Check sheet for the modelled part. Datum: model origin and axes. Units: mm. Face numbers are marked on the shaded views. Coordinates: 2 decimals unless noted, no trailing zeros. Write each loop counter-clockwise with the first axis right and the second up, starting at its lowest first coordinate (ties: lowest second). Pieces come first, ordered by that corner, then holes. Notation, with made-up numbers: M 15,33 L 47,33 A21 cw 47,44 Z; hole C 26,82 d7. An arc over 180 degrees is marked long. Answer as CSV lines item,"result". Start each with the question number.
Q1. Sectioned sample at A-A, the plane y = 12. Record the cut outline in (x, z).
Q2. Mould release check, pull along X, two halves, no side actions. Record for the marked faces 1 and 2: pulls with the +X half, pulls with the -X half, needs draft (parallel to the pull), parting line crosses it, or undercut.
Q3. Sectioned sample at C-C, the plane y = 61. Record the cut outline in (x, z), then the cut area to 3 significant figures.
Q4. Sectioned sample at D-D, the plane z = 18. Record the cut outline in (x, y).
Q5. Depth check by flat-ended pin: pin 1 Ø4.5 at (y, z) = (80.98, 9.12) entering from -X; pin 2 Ø0.5 at (x, y) = (1, 47.5) entering from -Z; pin 3 Ø3 at (x, z) = (-2.5, 9.5) entering from -Y; pin 4 Ø0.8 at (x, z) = (1, 6) entering from -Y. Enter the tip coordinate at first touch or a pass-through.
Q6. Thickness scan on line 1 along Y through (x, z) = (0.55, 10.5); line 2 along X through (y, z) = (62, 13.25); line 3 along Y through (x, z) = (0.7, 3.25). Record the ranges inside material, lowest first. Write a range as from..to.
Q7. Sectioned sample at B-B, the plane z = 4.75. Record the cut outline in (x, y), then the cut area to 3 significant figures.
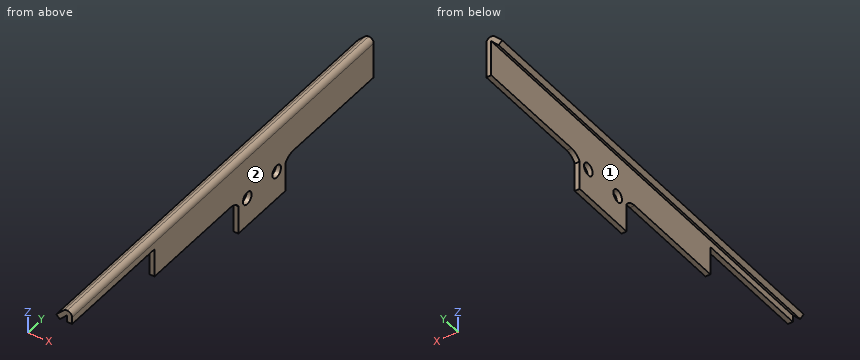
from build123d import *

# Parameters (mm, degrees)
F0_W      = 139.446
F0_H      = 24.0284
F1_DEPTH  = 1.5748
F2_R      = 2.5273
F2_R_2    = 1.9812
F3_DEPTH  = 25.4
F4_W      = 76.8604
F4_H      = 9.1186
F4_W_2    = 40.894
F5_DEPTH  = 25.4
F7_DEPTH  = 25.4
F9_DEPTH  = 139.447
F10_DEPTH = 139.446
F11_R     = 2.5273
F12_DEPTH = 25.4
F14_DEPTH = 1.5748
F15_DEPTH = 25.4


# Not quite as in the source:
# - ends of sketch curves that miss each other by under 0.0002 mm in the source are joined


with BuildPart() as f1:
    # F0 (on Right) → F1 (new body)
    with BuildSketch(Plane.YZ):
        with Locations((69.723, 12.0142)):
            Rectangle(F0_W, F0_H)
    extrude(amount=F1_DEPTH)

    # F2 (on face) → F3 (cut)
    with BuildSketch(Plane.YZ.offset(1.5748)):
        with Locations((7.9502, 14.6812)):
            Circle(F2_R)
        with Locations((80.9752, 9.1186)):
            Circle(F2_R_2)
        with Locations((94.5642, 9.1186)):
            Circle(F2_R_2)
    extrude(amount=-F3_DEPTH, mode=Mode.SUBTRACT)

    # F4 (on face) → F5 (cut)
    with BuildSketch(Plane.YZ.offset(1.5748)):
        with Locations((38.4302, 4.5593)):
            Rectangle(F4_W, F4_H)
        with Locations((118.999, 4.5593)):
            Rectangle(F4_W_2, F4_H)
    extrude(amount=-F5_DEPTH, mode=Mode.SUBTRACT)

    # F6 (on face) → F7 (cut)
    with BuildSketch(Plane.YZ.offset(1.5748)):
        with BuildLine():
            ThreePointArc((102.3057040906, 11.0998), (104.4279345117, 10.5741090514), (106.0594081813, 9.1186))
            Line((106.0594081813, 9.1186), (139.446, 9.1186))
            Line((139.446, 9.1186), (139.446, 11.0998))
            Line((139.446, 11.0998), (102.3057040906, 11.0998))
        make_face()
        with BuildLine():
            Line((98.552, 9.1186), (106.0594081813, 9.1186))
            ThreePointArc((106.0594081813, 9.1186), (104.4279345117, 10.5741090514), (102.3057040906, 11.0998))
            ThreePointArc((102.3057040906, 11.0998), (100.1834736696, 10.5741090514), (98.552, 9.1186))
        make_face()
        with BuildLine():
            ThreePointArc((25.0643040906, 9.1186), (23.4328304559, 10.574109033), (21.3106000788, 11.0998))
            ThreePointArc((21.3106000788, 11.0998), (19.1883696138, 10.5741090698), (17.5568959094, 9.1186))
            Line((17.5568959094, 9.1186), (25.0643040906, 9.1186))
        make_face()
        with BuildLine():
            ThreePointArc((69.3529918187, 9.1186), (70.9844654883, 10.5741090514), (73.1066959094, 11.0998))
            Line((73.1066959094, 11.0998), (21.3106000788, 11.0998))
            ThreePointArc((21.3106000788, 11.0998), (23.4328304559, 10.574109033), (25.0643040906, 9.1186))
            Line((25.0643040906, 9.1186), (69.3529918187, 9.1186))
        make_face()
        with BuildLine():
            ThreePointArc((76.8604, 9.1186), (75.2289263304, 10.5741090514), (73.1066959094, 11.0998))
            ThreePointArc((73.1066959094, 11.0998), (70.9844654883, 10.5741090514), (69.3529918187, 9.1186))
            Line((69.3529918187, 9.1186), (76.8604, 9.1186))
        make_face()
    extrude(amount=-F7_DEPTH, mode=Mode.SUBTRACT)

    # F8 (on face) → F9 (cut, through all)
    with BuildSketch(Plane.XZ):
        with BuildLine():
            Line((1.5748, 24.0284), (0, 24.0284))
            ThreePointArc((0, 24.0284), (1.1139794542, 23.562560882), (1.5748, 22.4465026135))
            Line((1.5748, 22.4465026135), (1.5748, 24.0284))
        make_face()
    extrude(amount=-F9_DEPTH, mode=Mode.SUBTRACT)

    # F8 (on face) → F10 (join)
    with BuildSketch(Plane.XZ):
        with BuildLine():
            Line((0, 24.0284), (0, 22.4536))
            Line((0, 22.4536), (0, 22.4465026135))
            Line((0, 22.4465026135), (1.5748, 22.4465026135))
            ThreePointArc((1.5748, 22.4465026135), (1.1139794542, 23.562560882), (0, 24.0284))
        make_face()
        with BuildLine():
            Line((-1.2264893587, 23.4542141594), (-0.0070973865, 22.4465026135))
            Line((-0.0070973865, 22.4465026135), (0, 22.4536))
            Line((0, 22.4536), (0, 24.0284))
            ThreePointArc((0, 24.0284), (-0.6777928151, 23.8791808689), (-1.2264893587, 23.4542141594))
        make_face()
        Polygon((-3.4544, 21.226303518), (-2.340848241, 20.112751759), (-0.0070973865, 22.4465026135), (-1.2264893587, 23.4542141594), align=None)
    extrude(amount=-F10_DEPTH)

    # F11 (on face) → F12 (cut)
    with BuildSketch(Plane(origin=(0, 0, 0), x_dir=(0, -1, 0), z_dir=(-1, 0, 0))):
        with BuildLine():
            Line((-17.5568959094, 9.1186), (0, 9.1186))
            Line((0, 9.1186), (0, 20.2311))
            Line((0, 20.2311), (-38.1, 20.2311))
            Line((-38.1, 20.2311), (-38.1, 11.0998))
            Line((-38.1, 11.0998), (-21.3106000788, 11.0998))
            ThreePointArc((-21.3106000788, 11.0998), (-19.1883696138, 10.5741090698), (-17.5568959094, 9.1186))
        make_face()
        with Locations((-7.9502, 14.6812)):
            Circle(F11_R, mode=Mode.SUBTRACT)
    extrude(amount=-F12_DEPTH, mode=Mode.SUBTRACT)


with BuildPart() as f14:
    # F13 (on Right) → F14 (new body, through all)
    with BuildSketch(Plane.YZ):
        with BuildLine():
            Line((38.1, 20.2311), (0, 20.2311))
            Line((0, 20.2311), (0, 0))
            Line((0, 0), (16.764, 0))
            Line((16.764, 0), (16.764, 6.5532))
            ThreePointArc((16.764, 6.5532), (18.0956683087, 9.7681316913), (21.3106, 11.0998))
            Line((21.3106, 11.0998), (38.1, 11.0998))
            Line((38.1, 11.0998), (38.1, 20.2311))
        make_face()
    extrude(amount=F14_DEPTH)

    # F2 (on face) → F15 (cut)
    with BuildSketch(Plane.YZ.offset(1.5748)):
        with Locations((7.9502, 14.6812)):
            Circle(F2_R)
    extrude(amount=-F15_DEPTH, mode=Mode.SUBTRACT)


solid = f1.part
Output:
1,outline,"M -3.45,21.23 L -2.34,20.11 L 0,22.45 L 0,20.23 L 1.57,20.23 L 1.57,22.45 A1.58 ccw 0,24.03 A1.58 ccw -1.23,23.45 Z"
2,face 1,"undercut"
2,face 2,"pulls with the +X half"
3,outline,"M -3.45,21.23 L -2.34,20.11 L 0,22.45 L 0,11.1 L 1.57,11.1 L 1.57,22.45 A1.58 ccw 0,24.03 A1.58 ccw -1.23,23.45 Z"
3,area,"26.0 mm^2"
4,outline,"M 0,38.1 L 1.57,38.1 L 1.57,139.45 L 0,139.45 Z"
5,pin 1,"stops at x = 0"
5,pin 2,"stops at z = 11.1"
5,pin 3,"passes through"
5,pin 4,"stops at y = 76.86"
6,line 1,"y = 75.36..79.56, 82.4..93.14, 95.98..100.05"
6,line 2,"x = 0..1.57"
6,line 3,"y = 76.86..98.55"
7,outline,"M 0,76.86 L 1.57,76.86 L 1.57,98.55 L 0,98.55 Z"
7,area,"34.2 mm^2"
